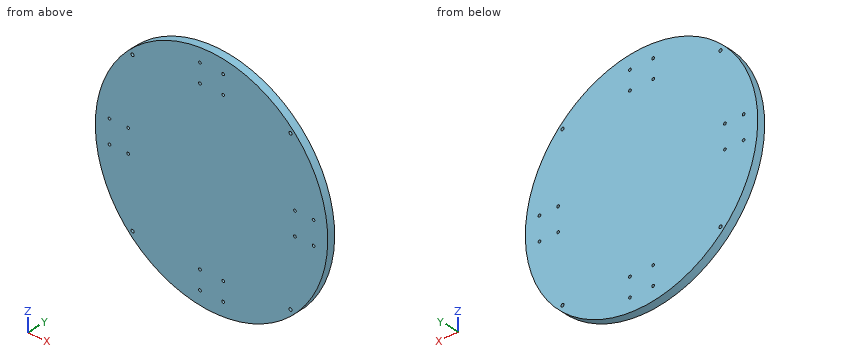
from build123d import *

# Parameters (mm, degrees)
SKETCH1_R           = 150
BOSS_EXTRUDE1_DEPTH = 10
SKETCH2_R           = 1.73
SKETCH2_R_2         = 2
CUT_EXTRUDE1_DEPTH  = 10


with BuildPart() as part:
    # Sketch1 → Boss-Extrude1 (new body)
    with BuildSketch(Plane(origin=(0, 0, 0), x_dir=(1, 0, 0), z_dir=(0, 1, 0))):
        with Locations(Location((0, 0, 0), (0, 0, 270))):
            Circle(SKETCH1_R)
    extrude(amount=BOSS_EXTRUDE1_DEPTH)

    # Sketch2 → Cut-Extrude1 (cut)
    with BuildSketch(Plane(origin=(0, 10, 0), x_dir=(1, 0, 0), z_dir=(0, 1, 0))):
        with Locations(Location((-14.945, 131.706442493, 0), (0, 0, 270))):
            Circle(SKETCH2_R)
        with Locations(Location((-14.945, 107.646442493, 0), (0, 0, 270))):
            Circle(SKETCH2_R)
        with Locations(Location((14.945, 107.646442493, 0), (0, 0, 90))):
            Circle(SKETCH2_R)
        with Locations(Location((14.945, 131.706442493, 0), (0, 0, 90))):
            Circle(SKETCH2_R)
        with Locations(Location((131.706442493, 14.945, 0), (0, 0, 270))):
            Circle(SKETCH2_R)
        with Locations(Location((131.706442493, -14.945, 0), (0, 0, 90))):
            Circle(SKETCH2_R)
        with Locations(Location((107.646442493, -14.945, 0), (0, 0, 90))):
            Circle(SKETCH2_R)
        with Locations(Location((107.646442493, 14.945, 0), (0, 0, 270))):
            Circle(SKETCH2_R)
        with Locations(Location((14.945, -131.706442493, 0), (0, 0, 270))):
            Circle(SKETCH2_R)
        with Locations(Location((-14.945, -131.706442493, 0), (0, 0, 90))):
            Circle(SKETCH2_R)
        with Locations(Location((-14.945, -107.646442493, 0), (0, 0, 90))):
            Circle(SKETCH2_R)
        with Locations(Location((14.945, -107.646442493, 0), (0, 0, 270))):
            Circle(SKETCH2_R)
        with Locations(Location((-131.706442493, -14.945, 0), (0, 0, 270))):
            Circle(SKETCH2_R)
        with Locations(Location((-131.706442493, 14.945, 0), (0, 0, 90))):
            Circle(SKETCH2_R)
        with Locations(Location((-107.646442493, 14.945, 0), (0, 0, 90))):
            Circle(SKETCH2_R)
        with Locations(Location((-107.646442493, -14.945, 0), (0, 0, 270))):
            Circle(SKETCH2_R)
        with Locations(Location((101.974532959, 101.974532959, 0), (0, 0, 270))):
            Circle(SKETCH2_R_2)
        with Locations(Location((101.974532959, -101.974532959, 0), (0, 0, 270))):
            Circle(SKETCH2_R_2)
        with Locations(Location((-101.974532959, -101.974532959, 0), (0, 0, 270))):
            Circle(SKETCH2_R_2)
        with Locations(Location((-101.974532959, 101.974532959, 0), (0, 0, 270))):
            Circle(SKETCH2_R_2)
    extrude(amount=-CUT_EXTRUDE1_DEPTH, mode=Mode.SUBTRACT)


solid = part.part
Check sheet for the modelled part. Datum: model origin and axes. Units: mm. Give positions to 0.01 mm unless a question says otherwise; leave off trailing zeros. Write each loop counter-clockwise with the first axis right and the second up, starting at its lowest first coordinate (ties: lowest second). Pieces come first, ordered by that corner, then holes. Notation, with made-up numbers: (51.5, 49.25) -> (90.5, 49.25) arc R14 ccw to (90.5, 75.25) -> close; hole circle Ø5 at (6.25, 79.25). An arc over 180 degrees is marked (long way). Use one line per item in the form item = value. Start each with the question number.
1. Thickness scan on line 1 along Z through (x, y) = (-107, 6.5); line 2 along X through (y, z) = (0.75, -107.5); line 3 along X through (y, z) = (9, 101.5). Record the ranges inside material, lowest first. Write a range as from..to.
2. Go/stop test with flat-tipped pins: P1, Ø2, axis at x = 14.94, z = -131.71, coming from the -Y side; P2, Ø1, axis at x = 27, y = 3, coming from the +Z side; P3, Ø4, axis at x = -66.5, y = 2.5, coming from the +Z side; P4, Ø1.5, axis at y = 9, z = 105, coming from the -X side. Record where each tip stops, or that it passes through.
3. Section check C-C (x = -28.5). Record the cut outline in (y, z), and give its area (3 significant figures).
4. Section check A-A (y = 5). Count the separate pieces of the cut face and the enclosed holes in it, and give its area (3 significant figures).
5. Section check B-B (z = 42). Record the cut outline in (x, y).
Conclusion:
q1.line_1 = -105.12..-16.55, -13.34..13.34, 16.55..105.12
q1.line_2 = -104.61..-16.67, -13.22..13.22, 16.67..104.61
q1.line_3 = -110.44..-103.92, -100.03..100.03, 103.92..110.44
q2.P1 = through
q2.P2 = 147.64
q2.P3 = 135.42
q2.P4 = -107.85
q3.outline = (0, -147.27) -> (10, -147.27) -> (10, 147.27) -> (0, 147.27) -> close
q3.area = 2,950 mm²
q4.separate_pieces = 1
q4.enclosed_holes = 20
q4.area = 70,500 mm²
q5.outline = (-144, 0) -> (144, 0) -> (144, 10) -> (-144, 10) -> close
